```python
from build123d import *

# Parameters (mm, degrees)
F0_R     = 11.25
F0_R_2   = 6.1
F0_R_3   = 4.125
F1_DEPTH = 2.54
F2_DEPTH = 4.25
F3_DEPTH = 1
F5_W     = 2.82376213
F5_H     = 0.5161568988
F5_W_2   = 0.7975271437
F5_H_2   = 2.7843180578
F5_H_3   = 2.6690037921
F5_H_4   = 1.2320959941
F5_H_5   = 1.4468301088
F5_H_6   = 1.1431314051
F6_DEPTH = 0.4318


# Not quite as in the source:
# - a fillet or chamfer that OpenCascade refuses, or shapes differently, is made with other operations: its cross-section is extruded or revolved along the edge and cut away or added


with BuildPart() as f1:
    # F0 (on Front) → F1 (new body)
    with BuildSketch(Plane.XZ):
        Circle(F0_R)
        Circle(F0_R_2, mode=Mode.SUBTRACT)
        Circle(F0_R_2)
        Circle(F0_R_3, mode=Mode.SUBTRACT)
        Circle(F0_R_3)
    extrude(amount=F1_DEPTH)

    # F0 (on Front) → F2 (join)
    with BuildSketch(Plane.XZ):
        Circle(F0_R_3)
    extrude(amount=-F2_DEPTH)

    # F0 (on Front) → F3 (join)
    with BuildSketch(Plane.XZ):
        Circle(F0_R_2)
        Circle(F0_R_3, mode=Mode.SUBTRACT)
    extrude(amount=-F3_DEPTH)

    # F4: fillet of radius 1.27 on 3 edges, made by hand

    # F4_s1 → F4_t2 (revolve, cut)
    with BuildSketch(Plane.XY):
        with BuildLine():
            ThreePointArc((6.1, 0), (5.6559015079, 0.7188882647), (4.8590326354, 1))
            Line((4.8590326354, 1), (6.1, 1))
            Line((6.1, 1), (6.1, 0))
        make_face()
    revolve(axis=Axis((0, 1, 0), (0, -1, 0)), mode=Mode.SUBTRACT)

    # F4_s3 → F4_t4 (revolve, cut)
    with BuildSketch(Plane.XY):
        with BuildLine():
            ThreePointArc((11.25, -1.27), (10.8780256121, -0.3719743879), (9.98, 0))
            Line((9.98, 0), (11.25, 0))
            Line((11.25, 0), (11.25, -1.27))
        make_face()
    revolve(axis=Axis((0, 0, 0), (0, -1, 0)), mode=Mode.SUBTRACT)

    # F4_s5 → F4_t6 (revolve, cut)
    with BuildSketch(Plane.XY):
        with BuildLine():
            ThreePointArc((11.25, -1.27), (10.8780256121, -2.1680256121), (9.98, -2.54))
            Line((9.98, -2.54), (11.25, -2.54))
            Line((11.25, -2.54), (11.25, -1.27))
        make_face()
    revolve(axis=Axis((0, -2.54, 0), (0, -1, 0)), mode=Mode.SUBTRACT)

    # F5 (on face) → F6 (join)
    with BuildSketch(Plane.XZ.offset(2.54)):
        with Locations((-5.6011655834, -0.2580784494)):
            Rectangle(F5_W, F5_H)
        Polygon((-2.7183012693, 5.0442311913), (-2.0541941821, 5.0442311913), (-3.3917573746, 7.5843841769), (-4.882786423, 7.5843841769), (-4.882786423, 6.7868568003), (-4.1892845184, 6.7868568003), (-4.1892845184, 5.0442311913), (-3.3917573746, 5.0442311913), (-3.3917573746, 6.2939338386), align=None)
        Polygon((-0.3677175585, 1.1431314051), (0, 1.1431314051), (-0.2914590528, 1.6966384), align=None)
        Polygon((3.3917573746, 5.0442311913), (4.1892845184, 5.0442311913), (4.1892845184, 6.7868568003), (4.882786423, 6.7868568003), (4.882786423, 7.5843841769), (3.3917573746, 7.5843841769), (2.0541941821, 5.0442311913), (2.7183012693, 5.0442311913), (3.3917573746, 6.2939338386), align=None)
        Polygon((-0.521645051, 5.0442311913), (0.521645051, 5.0442311913), (0.2444440033, 6.6919331439), (0.9331664045, 6.8078003193), (0.9331664045, 7.516650483), (0, 7.516650483), (-0.9331664045, 7.516650483), (-0.9331664045, 6.8078003193), (-0.2444440033, 6.6919331439), align=None)
        Polygon((0.6160256007, 1.1431314051), (1.1779463597, 1.1431314051), (1.0442581093, 1.9377834924), align=None)
        Polygon((0, 1.1431314051), (0.3677175585, 1.1431314051), (0.2914590528, 1.6966384), align=None)
        with BuildLine():
            ThreePointArc((6.1259130016, 3.8121351972), (7.4410236088, 2.4776333012), (6.1259130016, 1.1431314051))
            Line((6.1259130016, 1.1431314051), (4.1892845184, 1.1431314051))
            Line((4.1892845184, 1.1431314051), (4.1892845184, 0))
            Line((4.1892845184, 0), (8.4969736636, 0))
            ThreePointArc((8.4969736636, 0), (8.9127659298, 3.2748235651), (6.1259130016, 5.0442311913))
            Line((6.1259130016, 5.0442311913), (5.1765339449, 5.0442311913))
            Line((5.1765339449, 5.0442311913), (4.1892845184, 5.0442311913))
            Line((4.1892845184, 5.0442311913), (4.1892845184, 3.8121351972))
            Line((4.1892845184, 3.8121351972), (6.1259130016, 3.8121351972))
        make_face()
        Polygon((-3.3917573746, -5.4534515366), (-3.3917573746, -4.7473050654), (-4.1892845184, -4.7473050654), (-4.1892845184, -5.4534515366), (-4.882786423, -5.4534515366), (-4.882786423, -5.8025359176), (-2.9781798366, -5.8025359176), (-2.9781798366, -5.4534515366), align=None)
        Polygon((-0.8081396227, -5.8025359176), (-1.1792626465, -4.7473050654), (-2.1689236164, -4.7473050654), (-2.5400463492, -5.8025359176), align=None)
        Polygon((2.5400463492, -5.8025359176), (2.1689236164, -4.7473050654), (1.1792626465, -4.7473050654), (0.8081396227, -5.8025359176), align=None)
        Polygon((4.1892845184, -5.4534515366), (4.1892845184, -4.7473050654), (3.3917573746, -4.7473050654), (3.3917573746, -5.4534515366), (2.9781798366, -5.4534515366), (2.9781798366, -5.8025359176), (4.882786423, -5.8025359176), (4.882786423, -5.4534515366), align=None)
        with Locations((-3.7905209465, -1.9083159277)):
            Rectangle(F5_W_2, F5_H_2)
        with Locations((-3.7905209465, -0.2580784494)):
            Rectangle(F5_W_2, F5_H)
        with Locations((-3.7905209465, 2.4776333012)):
            Rectangle(F5_W_2, F5_H_3)
        with Locations((-3.7905209465, 4.4281831942)):
            Rectangle(F5_W_2, F5_H_4)
        Polygon((-0.3677175585, 1.1431314051), (-0.2914590528, 1.6966384), (-0.8927262809, 2.8384990261), (-1.0442581093, 1.9377834924), (-0.6160256007, 1.1431314051), align=None)
        Polygon((-1.0442581093, 1.9377834924), (-0.8927262809, 2.8384990261), (-1.4054118998, 3.8121351972), (-2.0543332675, 3.8121351972), align=None)
        Polygon((-0.2914590528, 1.6966384), (0, 3.8121351972), (-0.728926653, 3.8121351972), (-0.8927262809, 2.8384990261), align=None)
        Polygon((0.2914590528, 1.6966384), (0.8927262809, 2.8384990261), (0.728926653, 3.8121351972), (0, 3.8121351972), align=None)
        Polygon((0.6160256007, 1.1431314051), (1.0442581093, 1.9377834924), (0.8927262809, 2.8384990261), (0.2914590528, 1.6966384), (0.3677175585, 1.1431314051), align=None)
        Polygon((0, 0), (0.4182745639, 0.7761735704), (0.3677175585, 1.1431314051), (0, 1.1431314051), (-0.3677175585, 1.1431314051), (-0.4182745639, 0.7761735704), align=None)
        with Locations((3.7905209465, -1.9083159277)):
            Rectangle(F5_W_2, F5_H_2)
        with Locations((3.7905209465, -0.2580784494)):
            Rectangle(F5_W_2, F5_H)
        with Locations((3.7905209465, 2.4776333012)):
            Rectangle(F5_W_2, F5_H_3)
        with Locations((3.7905209465, 4.4281831942)):
            Rectangle(F5_W_2, F5_H_4)
        Polygon((1.0442581093, 1.9377834924), (2.0543332675, 3.8121351972), (1.4054118998, 3.8121351972), (0.8927262809, 2.8384990261), align=None)
        Polygon((-0.6160256007, 1.1431314051), (-0.4182745639, 0.7761735704), (-0.3677175585, 1.1431314051), align=None)
        Polygon((0.4182745639, 0.7761735704), (0.6160256007, 1.1431314051), (0.3677175585, 1.1431314051), align=None)
        Polygon((-1.4054118998, 3.8121351972), (-2.0541941821, 5.0442311913), (-2.7183012693, 5.0442311913), (-2.0543332675, 3.8121351972), align=None)
        Polygon((1.4054118998, 3.8121351972), (2.0543332675, 3.8121351972), (2.7183012693, 5.0442311913), (2.0541941821, 5.0442311913), align=None)
        Polygon((-8.0940451721, 0), (-7.0130466484, 0), (-7.0130466484, 1.1431314051), (-7.0130466484, 3.8121351972), (-4.1892845184, 3.8121351972), (-4.1892845184, 5.0442311913), (-7.7138240449, 5.0442311913), (-8.3028590307, 5.0442311913), (-8.3028590307, 4.5893052593), (-8.1096682698, 4.5893052593), align=None)
        Polygon((2.0543332675, 3.8121351972), (3.3917573746, 3.8121351972), (3.3917573746, 5.0442311913), (2.7183012693, 5.0442311913), align=None)
        with Locations((-3.7905209465, -4.023890011)):
            Rectangle(F5_W_2, F5_H_5)
        Polygon((-2.0543332675, 3.8121351972), (-2.7183012693, 5.0442311913), (-3.3917573746, 5.0442311913), (-3.3917573746, 3.8121351972), align=None)
        Polygon((-0.728926653, 3.8121351972), (-0.521645051, 5.0442311913), (-2.0541941821, 5.0442311913), (-1.4054118998, 3.8121351972), align=None)
        Polygon((0, 3.8121351972), (0.728926653, 3.8121351972), (0.521645051, 5.0442311913), (-0.521645051, 5.0442311913), (-0.728926653, 3.8121351972), align=None)
        Polygon((0.728926653, 3.8121351972), (1.4054118998, 3.8121351972), (2.0541941821, 5.0442311913), (0.521645051, 5.0442311913), align=None)
        Polygon((-1.1779463597, 1.1431314051), (-0.6160256007, 1.1431314051), (-1.0442581093, 1.9377834924), align=None)
        Polygon((1.4570966365, -0.5161568988), (1.370261009, 0), (0.5252105866, 0), (0.5963232449, -0.5161568988), align=None)
        Polygon((3.3917573746, -0.5161568988), (3.3917573746, 0), (1.370261009, 0), (1.4570966365, -0.5161568988), align=None)
        Polygon((-3.3917573746, -0.5161568988), (-1.4570966365, -0.5161568988), (-1.370261009, 0), (-3.3917573746, 0), align=None)
        Polygon((-1.4570966365, -0.5161568988), (-0.5963232449, -0.5161568988), (-0.5252105866, 0), (-1.370261009, 0), align=None)
        Polygon((-0.9799280345, -3.3004749566), (-0.5963232449, -0.5161568988), (-1.4570966365, -0.5161568988), (-1.9255162324, -3.3004749566), align=None)
        Polygon((1.9255162324, -3.3004749566), (1.4570966365, -0.5161568988), (0.5963232449, -0.5161568988), (0.9799280345, -3.3004749566), align=None)
        Polygon((2.1689236164, -4.7473050654), (1.9255162324, -3.3004749566), (0.9799280345, -3.3004749566), (1.1792626465, -4.7473050654), align=None)
        Polygon((3.3917573746, -4.7473050654), (3.3917573746, -3.3004749566), (1.9255162324, -3.3004749566), (2.1689236164, -4.7473050654), align=None)
        with Locations((3.7905209465, -4.023890011)):
            Rectangle(F5_W_2, F5_H_5)
        Polygon((-1.1792626465, -4.7473050654), (-0.9799280345, -3.3004749566), (-1.9255162324, -3.3004749566), (-2.1689236164, -4.7473050654), align=None)
        Polygon((-2.1689236164, -4.7473050654), (-1.9255162324, -3.3004749566), (-3.3917573746, -3.3004749566), (-3.3917573746, -4.7473050654), align=None)
        Polygon((1.1792626465, -4.7473050654), (0.9799280345, -3.3004749566), (-0.9799280345, -3.3004749566), (-1.1792626465, -4.7473050654), align=None)
        Polygon((0.5963232449, -0.5161568988), (0.5252105866, 0), (0, 0), (-0.5252105866, 0), (-0.5963232449, -0.5161568988), align=None)
        with Locations((-5.6011655834, 0.5715657026)):
            Rectangle(F5_W, F5_H_6)
        with Locations((-3.7905209465, 0.5715657026)):
            Rectangle(F5_W_2, F5_H_6)
        Polygon((-3.3917573746, 0), (-1.370261009, 0), (-1.1779463597, 1.1431314051), (-3.3917573746, 1.1431314051), align=None)
        Polygon((-0.5252105866, 0), (-0.4182745639, 0.7761735704), (-0.6160256007, 1.1431314051), (-1.1779463597, 1.1431314051), (-1.370261009, 0), align=None)
        Polygon((-0.5252105866, 0), (0, 0), (-0.4182745639, 0.7761735704), align=None)
        Polygon((0, 0), (0.5252105866, 0), (0.4182745639, 0.7761735704), align=None)
        Polygon((1.370261009, 0), (1.1779463597, 1.1431314051), (0.6160256007, 1.1431314051), (0.4182745639, 0.7761735704), (0.5252105866, 0), align=None)
        Polygon((3.3917573746, 0), (3.3917573746, 1.1431314051), (1.1779463597, 1.1431314051), (1.370261009, 0), align=None)
        with Locations((3.7905209465, 0.5715657026)):
            Rectangle(F5_W_2, F5_H_6)
        with BuildLine():
            Line((8.4969736636, 0), (4.1892845184, 0))
            Line((4.1892845184, 0), (4.1892845184, -0.5161568988))
            Line((4.1892845184, -0.5161568988), (6.1259130016, -0.5161568988))
            ThreePointArc((6.1259130016, -0.5161568988), (7.1544234466, -1.9083159277), (6.1259130016, -3.3004749566))
            Line((6.1259130016, -3.3004749566), (4.1892845184, -3.3004749566))
            Line((4.1892845184, -3.3004749566), (4.1892845184, -4.7473050654))
            Line((4.1892845184, -4.7473050654), (6.1259130016, -4.7473050654))
            ThreePointArc((6.1259130016, -4.7473050654), (8.7791579039, -3.106708495), (8.4969736636, 0))
        make_face()
        Polygon((-4.1892845184, -4.7473050654), (-4.1892845184, -3.3004749566), (-7.0130466484, -3.3004749566), (-7.0130466484, -0.5161568988), (-7.0130466484, 0), (-8.0940451721, 0), (-8.0794328824, -4.2923791334), (-8.2726236433, -4.2923791334), (-8.2726236433, -4.7473050654), (-7.7138240449, -4.7473050654), (-7.6835886575, -4.7473050654), align=None)
    extrude(amount=F6_DEPTH)


solid = f1.part
```
Input: part model. Units: mm. Frame: model coordinates. A direction names the side the tool comes from. Give positions to 0.01 mm unless a question says otherwise; leave off trailing zeros. Order: outer loops, then holes, each group sorted by start corner. A loop starts at its lowest first (then second) coordinate and runs counter-clockwise, first axis right, second up. Notation, with made-up numbers: (-2.5, 28.5) - (48.5, 28.5) arc R12 cw to (48.5, 44.5) - close; hole circle Ø4 at (-39, 61). An arc over 180 degrees is marked (long way). One line per item, written item: value.
1. Cut plane A-A, the plane y = 3.25. Output: boundary loops of the cut face in (x, z) (3 decimals), and give its area (3 significant figures).
Determined:
outline: circle Ø8.25 at (0, 0)
area: 53.5 mm2
2. Reachability of faces 1 (the face through (6, -2.54, 2)), 2 (the face through (-2, 1, -4)), 3 (the face through (8.933, -2.753, 3.231)) from +Z, -Z, +X, -X, +Y, -Y: full face, straight path, thin tool, end or side. Return the list, or none.
Determined:
face 1: -Y
face 2: +Y
face 3: +X, -Y
3. Pin query (flat end, axial travel): pin 1 Ø4 at (y, z) = (2.5, -1) entering from -X; pin 2 Ø1.5 at (x, y) = (7, -1.5) entering from +Z; pin 3 Ø0.5 at (y, z) = (-2.5, 5.5) entering from -X. Return the tip coordinate at first contact, or that it passes through.
Determined:
pin 1: x = -5.81
pin 2: z = 9.34
pin 3: x = -9.31
4. Line query: probe 1 along Y at (x, z) = (-3.5, -8.5); probe 2 along Y at (x, z) = (0.5, -5.25); probe 3 along Z at (x, y) = (2, 4). Output: solid intervals per line, ascending.
Determined:
probe 1: -2.54 to 0
probe 2: -2.54 to 0.93
probe 3: -3.61 to 3.61
5. Draft query along Z for faces 4 (the face through (-6, -2.54, 2)), 5 (the face through (3.8, 2.6, -1.6)), 6 (the face through (2.73, -2.75, 6.33)). Return one class per face: released by +Z, released by -Z, zero draft, split by the parting line, or undercut.
Determined:
face 4: undercut
face 5: split by the parting line
face 6: released by +Z
